Input: part model. Units: mm. Frame: model coordinates. Face numbers are marked on the shaded views. Coordinates: 2 decimals unless noted, no trailing zeros. Order: outer loops, then holes, each group sorted by start corner. A loop starts at its lowest first (then second) coordinate and runs counter-clockwise, first axis right, second up. Notation, with made-up numbers: (32, 5) -> (39, 5) arc R25 ccw to (39, 20) -> close; hole circle Ø9 at (61.25, -25.75). An arc over 180 degrees is marked (long way). Write each question's results on one line, items separated by ' | '.
```python
from build123d import *

# Parameters (mm, degrees)
SKETCH1_R           = 9.5
BOSS_EXTRUDE1_DEPTH = 5
SKETCH2_R           = 1.575
SKETCH2_R_2         = 2
CUT_EXTRUDE1_DEPTH  = 5


with BuildPart() as part:
    # Sketch1 → Boss-Extrude1 (new body)
    with BuildSketch(Plane(origin=(0, 0, 0), x_dir=(1, 0, 0), z_dir=(0, 1, 0))):
        Circle(SKETCH1_R)
    extrude(amount=BOSS_EXTRUDE1_DEPTH)

    # Sketch2 → Cut-Extrude1 (cut)
    with BuildSketch(Plane(origin=(0, 5, 0), x_dir=(1, 0, 0), z_dir=(0, 1, 0))):
        with Locations((0, 6.35)):
            Circle(SKETCH2_R)
        with Locations((6.35, 0)):
            Circle(SKETCH2_R)
        with Locations((0, -6.35)):
            Circle(SKETCH2_R)
        with Locations((-6.35, 0)):
            Circle(SKETCH2_R)
        Circle(SKETCH2_R_2)
    extrude(amount=-CUT_EXTRUDE1_DEPTH, mode=Mode.SUBTRACT)


solid = part.part
```
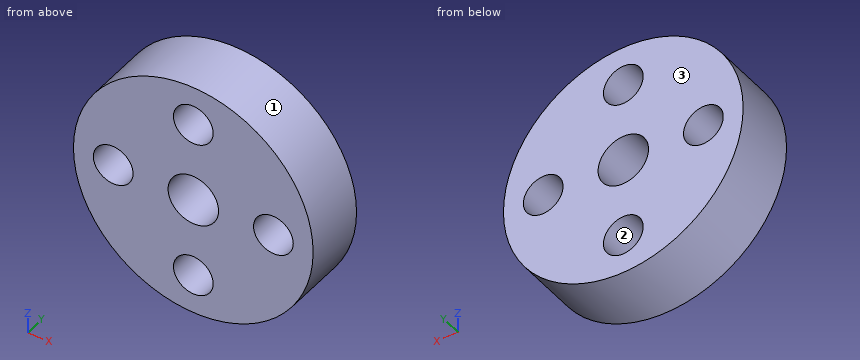
(1) Line query: line 1 along X through (y, z) = (2.65, 0) (3 decimals); line 2 along Z through (x, y) = (-0.5, 1.3). Output: solid intervals per line, ascending. Write a range as from..to.
Return value:
line 1: -9.5..-7.925, -4.775..-2, 2..4.775, 7.925..9.5 | line 2: -9.49..-7.84, -4.86..-1.94, 1.94..4.86, 7.84..9.49
(2) Cut plane D-D, the plane z = -5.25. Return loops of the section in (x, y), plus the area to 3 significant figures.
Return value:
outline: (-7.92, 0) -> (-1.13, 0) -> (-1.13, 5) -> (-7.92, 5) -> close; (1.13, 0) -> (7.92, 0) -> (7.92, 5) -> (1.13, 5) -> close | area: 67.9 mm2
(3) Pin query (flat end, axial travel): P1, Ø1.9, axis at x = 0, z = 6.35, coming from the -Y side; P2, Ø2, axis at y = 1.5, z = 5, coming from the -X side; P3, Ø1.5, axis at x = -1.5, y = 1, coming from the -Z side. Return the tip coordinate at first contact, or that it passes through.
Return value:
P1: through | P2: x = -8.62 | P3: z = -9.47
(4) Mould query, pull axis Z, two halves, no side actions, for the marked faces 1, 2 and 3. Classes: +Z half, -Z half, draft (parallel to the pull), parting line (faces both ways), or undercut.
Return value:
face 1: parting line | face 2: undercut | face 3: draft
(5) Cut plane A-A, the plane z = 0. Return loops of the section in (x, y) (3 decimals).
Return value:
outline: (-9.5, 0) -> (-7.925, 0) -> (-7.925, 5) -> (-9.5, 5) -> close; (-4.775, 0) -> (-2, 0) -> (-2, 5) -> (-4.775, 5) -> close; (2, 0) -> (4.775, 0) -> (4.775, 5) -> (2, 5) -> close; (7.925, 0) -> (9.5, 0) -> (9.5, 5) -> (7.925, 5) -> close
(6) Cut plane B-B, the plane x = 0. Return loops of the section in (y, z) (3 decimals).
Return value:
outline: (0, -9.5) -> (5, -9.5) -> (5, -7.925) -> (0, -7.925) -> close; (0, -4.775) -> (5, -4.775) -> (5, -2) -> (0, -2) -> close; (0, 2) -> (5, 2) -> (5, 4.775) -> (0, 4.775) -> close; (0, 7.925) -> (5, 7.925) -> (5, 9.5) -> (0, 9.5) -> close
(7) Cut plane C-C, the plane y = 1.25. Return loops of the section in (x, z) (3 decimals).
Return value:
outline: circle Ø19 at (0, 0); hole circle Ø3.15 at (-6.35, 0); hole circle Ø4 at (0, 0); hole circle Ø3.15 at (0, -6.35); hole circle Ø3.15 at (0, 6.35); hole circle Ø3.15 at (6.35, 0)
